from build123d import *

# Parameters (mm, degrees)
SKETCH1_W           = 111.76
SKETCH1_H           = 60.96
BOSS_EXTRUDE1_DEPTH = 5.08
FILLET1_R           = 5.08
CUT_EXTRUDE1_REACH  = 129.406
SKETCH3_R           = 2.794
SKETCH3_R_2         = 3.302
SKETCH5_W           = 10.16
SKETCH5_H           = 60.96
BOSS_EXTRUDE2_DEPTH = 5.08
FILLET2_R           = 5.08
SKETCH2_W           = 10.16
SKETCH2_H           = 10.16
SKETCH2_H_2         = 5.08
BOSS_EXTRUDE5_DEPTH = 25.4
FILLET9_R           = 2.286
FILLET10_R          = 5.08
SKETCH6_R           = 6.996125679
BOSS_EXTRUDE6_DEPTH = 5.08


with BuildPart() as part:
    # Sketch1 → Boss-Extrude1 (new body)
    with BuildSketch(Plane(origin=(0, 0, 0), x_dir=(1, 0, 0), z_dir=(0, 1, 0))):
        with Locations((55.88, 30.48)):
            Rectangle(SKETCH1_W, SKETCH1_H)
    extrude(amount=BOSS_EXTRUDE1_DEPTH)

    # Fillet1
    fillet1_edges = [part.edges().sort_by_distance(p)[0] for p in [
        (0, 2.54, -60.96),
        (111.76, 2.54, -60.96),
        (111.76, 2.54, 0),
        (0, 2.54, 0),
    ]]
    fillet(fillet1_edges, radius=FILLET1_R)

    # Sketch3 → Cut-Extrude1 (cut, up to next)
    with BuildSketch(Plane.XZ, mode=Mode.PRIVATE) as cut_extrude1_sk1:
        with Locations(Location((20.32, -17.78, 0), (0, 0, 270))):
            Circle(SKETCH3_R)
    cut_extrude1_tool1 = extrude(cut_extrude1_sk1.sketch, amount=-CUT_EXTRUDE1_REACH, mode=Mode.PRIVATE) & part.part
    # Sketch3 → Cut-Extrude1 (cut, up to next)
    with BuildSketch(Plane.XZ, mode=Mode.PRIVATE) as cut_extrude1_sk2:
        with Locations(Location((20.32, -43.18, 0), (0, 0, 270))):
            Circle(SKETCH3_R)
    cut_extrude1_tool2 = extrude(cut_extrude1_sk2.sketch, amount=-CUT_EXTRUDE1_REACH, mode=Mode.PRIVATE) & part.part
    # Sketch3 → Cut-Extrude1 (cut, up to next)
    with BuildSketch(Plane.XZ, mode=Mode.PRIVATE) as cut_extrude1_sk3:
        with Locations(Location((30.48, -30.48, 0), (0, 0, 270))):
            Circle(SKETCH3_R_2)
    cut_extrude1_tool3 = extrude(cut_extrude1_sk3.sketch, amount=-CUT_EXTRUDE1_REACH, mode=Mode.PRIVATE) & part.part
    add(cut_extrude1_tool1.solids().sort_by_distance((20.32, 0, -17.78))[0], mode=Mode.SUBTRACT)
    add(cut_extrude1_tool2.solids().sort_by_distance((20.32, 0, -43.18))[0], mode=Mode.SUBTRACT)
    add(cut_extrude1_tool3.solids().sort_by_distance((30.48, 0, -30.48))[0], mode=Mode.SUBTRACT)

    # Sketch5 → Boss-Extrude2 (add)
    with BuildSketch(Plane.XZ):
        with Locations((111.76, -30.48)):
            Rectangle(SKETCH5_W, SKETCH5_H)
    extrude(amount=-BOSS_EXTRUDE2_DEPTH)

    # Fillet2
    fillet2_edges = [part.edges().sort_by_distance(p)[0] for p in [
        (116.84, 2.54, 0),
        (116.84, 2.54, -60.96),
    ]]
    fillet(fillet2_edges, radius=FILLET2_R)

    # Sketch2 → Boss-Extrude5 (add)
    with BuildSketch(Plane(origin=(0, 5.08, 0), x_dir=(1, 0, 0), z_dir=(0, 1, 0))):
        with Locations((7.874, 53.086)):
            Rectangle(SKETCH2_W, SKETCH2_H)
        with Locations((7.874, 7.874)):
            Rectangle(SKETCH2_W, SKETCH2_H)
        with Locations((108.966, 55.626)):
            Rectangle(SKETCH2_W, SKETCH2_H_2)
        with Locations((108.966, 5.334)):
            Rectangle(SKETCH2_W, SKETCH2_H_2)
    extrude(amount=BOSS_EXTRUDE5_DEPTH)

    # Fillet9
    fillet9_edges = [part.edges().sort_by_distance(p)[0] for p in [
        (103.886, 17.78, -7.874),
        (114.046, 17.78, -2.794),
        (2.794, 17.78, -2.794),
        (2.794, 17.78, -58.166),
        (103.886, 17.78, -53.086),
        (114.046, 17.78, -58.166),
    ]]
    fillet(fillet9_edges, radius=FILLET9_R)

    # Fillet10
    fillet10_edges = [part.edges().sort_by_distance(p)[0] for p in [
        (12.954, 17.78, -12.954),
        (12.954, 17.78, -48.006),
    ]]
    fillet(fillet10_edges, radius=FILLET10_R)

    # Sketch6 → Boss-Extrude6 (add)
    with BuildSketch(Plane(origin=(0, 5.08, 0), x_dir=(1, 0, 0), z_dir=(0, 1, 0))):
        with Locations((30.48, 30.48)):
            Circle(SKETCH6_R)
    extrude(amount=-BOSS_EXTRUDE6_DEPTH)


solid = part.part
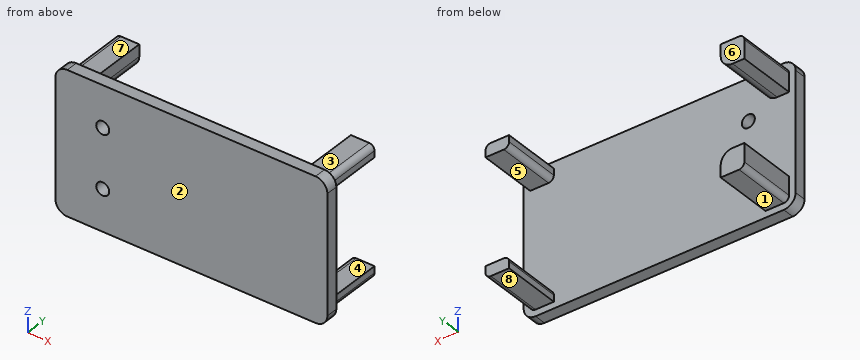
Could you check a few things on this model? Use its own coordinates, in mm. Face numbers are marked on the shaded views. A direction names the side the tool comes from. Give positions to 0.01 mm unless a question says otherwise; leave off trailing zeros. Order: outer loops, then holes, each group sorted by start corner. A loop starts at its lowest first (then second) coordinate and runs counter-clockwise, first axis right, second up. Notation, with made-up numbers: (-34, 20) -> (-19, 20) arc R15 ccw to (-19, 47) -> close; hole circle Ø11 at (57.5, 48.5). An arc over 180 degrees is marked (long way). Answer in a Markdown table with one row per item. Add a question column.
Item 1: I'm going to push flat-ended pins straight in: P1, Ø4, axis at y = 19.5, z = -5.5, coming from the +X side; P2, Ø1.4, axis at y = 13.5, z = -56, coming from the -X side; P3, Ø5.5, axis at x = 5.5, y = 16.5, coming from the +Z side. Where does each tip first touch, or does it pass through?
Item 2: Imagine slicing it at C-C (x = 20.32). List the corners of the cut face in (y, z) for me.
Item 3: Imagine slicing it at D-D (z = -39). List the corners of the cut face in (x, y) for me, and give its area (3 significant figures).
Item 4: For the marked faces 1, 2, 3 and 4, which set-ups out of +Z, -Z, +X, -X, +Y, -Y let a thin tool reach every point of the face, with its end or its side?
Item 5: Please list where these lines run through material, in increasing order: probe 1 along Z at (x, y) = (20, 2); probe 2 along X at (y, z) = (3.9, -43.18); probe 3 along X at (y, z) = (28, -5.5).
Item 6: We'd pull the mould along Z, two halves only. Please class the marked faces 5, 6, 7 and 8: pulls with the +Z half, pulls with the -Z half, needs draft (parallel to the pull), parting line crosses it, or undercut.
Item 7: Imagine slicing it at B-B (z = -17.78). List the corners of the cut face in (x, y) for me.
Item 8: Imagine slicing it at A-A (y = 9). List the corners of the cut face in (x, z) for me, and give its area (3 significant figures).
Result:
| question | item | result |
|---|---|---|
| 1 | P1 | x = 114.05 |
| 1 | P2 | x = 2.79 |
| 1 | P3 | z = -2.79 |
| 2 | outline | (0, -60.96) -> (5.08, -60.96) -> (5.08, -45.97) -> (0, -45.97) -> close; (0, -40.39) -> (5.08, -40.39) -> (5.08, -20.57) -> (0, -20.57) -> close; (0, -14.99) -> (5.08, -14.99) -> (5.08, 0) -> (0, 0) -> close |
| 3 | outline | (0, 0) -> (116.84, 0) -> (116.84, 5.08) -> (0, 5.08) -> close |
| 3 | area | 594 mm2 |
| 4 | face 1 | -Z, +X, -X, +Y |
| 4 | face 2 | +Z, -Z, +X, -X, -Y |
| 4 | face 3 | +Z, +X, -X, +Y |
| 4 | face 4 | +X, +Y |
| 5 | probe 1 | -60.96 to -45.96, -40.4 to -20.56, -15 to 0 |
| 5 | probe 2 | 0 to 17.53, 23.11 to 116.84 |
| 5 | probe 3 | 2.79 to 12.95, 103.89 to 114.05 |
| 6 | face 5 | undercut |
| 6 | face 6 | needs draft |
| 6 | face 7 | pulls with the +Z half |
| 6 | face 8 | pulls with the -Z half |
| 7 | outline | (0, 0) -> (17.53, 0) -> (17.53, 5.08) -> (0, 5.08) -> close; (23.11, 0) -> (116.84, 0) -> (116.84, 5.08) -> (23.11, 5.08) -> close |
| 8 | outline | (2.79, -55.88) arc R2.29 ccw to (5.08, -58.17) -> (12.95, -58.17) -> (12.95, -53.09) arc R5.08 ccw to (7.87, -48.01) -> (2.79, -48.01) -> close; (2.79, -12.95) -> (7.87, -12.95) arc R5.08 ccw to (12.95, -7.87) -> (12.95, -2.79) -> (5.08, -2.79) arc R2.29 ccw to (2.79, -5.08) -> close; (103.89, -58.17) -> (111.76, -58.17) arc R2.29 ccw to (114.05, -55.88) -> (114.05, -53.09) -> (106.17, -53.09) arc R2.29 ccw to (103.89, -55.37) -> close; (103.89, -5.59) arc R2.29 ccw to (106.17, -7.87) -> (114.05, -7.87) -> (114.05, -5.08) arc R2.29 ccw to (111.76, -2.79) -> (103.89, -2.79) -> close |
| 8 | area | 292 mm2 |
